Part model, mm, in its own coordinate system. A direction names the side the tool comes from. Coordinates: 2 decimals unless noted, no trailing zeros. Write each loop counter-clockwise with the first axis right and the second up, starting at its lowest first coordinate (ties: lowest second). Pieces come first, ordered by that corner, then holes. Notation, with made-up numbers: M 34,-39.75 L 74,-39.75 A29 cw 74,-10.75 Z; hole C 63.5,5 d1. An arc over 180 degrees is marked long. Use a Markdown table: item, result. Add a question column.
Q1. Slice it at C-C on y = -59. Write the cut outline in (x, z).
Q2. Tool access for faces 1 (the flat face through (36, -97, -12)), 2 (the cylindrical face through (-4.88, -51.88, 37.18)): list every direction of +Z, -Z, +X, -X, +Y, -Y with a clear straight run to the whole face (end or side of a thin tool).
Q3. Wall check: L1, parallel to Z at x = 0, y = -36; L2, parallel to Y at x = 26.5, z = 4; L3, parallel to X at y = -22, z = -4. Give the ranges that are in metal, low to high. Write a range as from..to.
Q4. Pin check, flat tips, straight feed: pin 1 Ø3 at (y, z) = (-47, 18) entering from -X; pin 2 Ø8 at (x, z) = (32.5, 16.5) entering from +Y; pin 3 Ø4 at (y, z) = (-55, 16.5) entering from -X; pin 4 Ø10 at (x, y) = (12, -69) entering from +Z. Stop position of each tip, or through.
Q5. Slice it at A-A on z = 0. Write the cut outline in (x, y).
Q6. Slice it at B-B on x = 0. Write the cut outline in (y, z), then the cut area to 3 significant figures.
Q7. Mould opens along Z. For faces 3 (the flat face through (-1, -8, 1)), 4 (the cylindrical face through (39.584, -47.835, 12.465)), 5 (the flat face through (-1, 0, 1)) say: released by +Z, released by -Z, zero draft, split by the parting line, or undercut.
from build123d import *

# Parameters (mm, degrees)
F0_R     = 41.5
F0_R_2   = 37.5
F1_DEPTH = 97
F2_DEPTH = 8
F3_SIZE  = 1


with BuildPart() as f1:
    # F0 (on Front) → F1 (new body)
    with BuildSketch(Plane.XZ):
        Circle(F0_R)
        Circle(F0_R_2, mode=Mode.SUBTRACT)
    extrude(amount=F1_DEPTH)

    # F0 (on Front) → F2 (join)
    with BuildSketch(Plane.XZ):
        Circle(F0_R_2)
    extrude(amount=F2_DEPTH)

    # F3
    f3_edges = [f1.edges().sort_by_distance(p)[0] for p in [
        (41.5, -48.5, 0),
        (-41.5, 0, 0),
        (-41.5, -97, 0),
    ]]
    chamfer(f3_edges, length=F3_SIZE)


solid = f1.part
Recorded:
| question | item | result |
|---|---|---|
| 1 | outline | C 0,0 d83; hole C 0,0 d75 |
| 2 | face 1 | +Z, -Z, +X, -X, -Y |
| 2 | face 2 | -Y |
| 3 | L1 | -41.5..-37.5, 37.5..41.5 |
| 3 | L2 | -8..0 |
| 3 | L3 | -41.31..-37.29, 37.29..41.31 |
| 4 | pin 1 | x = -38.08 |
| 4 | pin 2 | y = 0 |
| 4 | pin 3 | x = -38.88 |
| 4 | pin 4 | z = 40.91 |
| 5 | outline | M -41.5,-96 L -40.5,-97 L -37.5,-97 L -37.5,-8 L 37.5,-8 L 37.5,-97 L 40.5,-97 L 41.5,-96 L 41.5,-1 L 40.5,0 L -40.5,0 L -41.5,-1 Z |
| 6 | outline | M -97,-40.5 L -96,-41.5 L -1,-41.5 L 0,-40.5 L 0,40.5 L -1,41.5 L -96,41.5 L -97,40.5 L -97,37.5 L -8,37.5 L -8,-37.5 L -97,-37.5 Z |
| 6 | area | 1,370 mm² |
| 7 | face 3 | undercut |
| 7 | face 4 | split by the parting line |
| 7 | face 5 | zero draft |
